The drawing under review shows one solid part. Ordinate dimensions are in mm from its lowest x, y, z. Round coordinates to 2 decimals unless told otherwise and drop trailing zeros. Write each loop counter-clockwise with the first axis right and the second up, starting at its lowest first coordinate (ties: lowest second). Pieces come first, ordered by that corner, then holes. Notation, with made-up numbers: (20, 27.5) - (53, 27.5) arc R4 ccw to (53, 33.5) - close; hole circle Ø10 at (61.25, 73). An arc over 180 degrees is marked (long way). Answer in a Markdown table with one row per item. Add a question column.
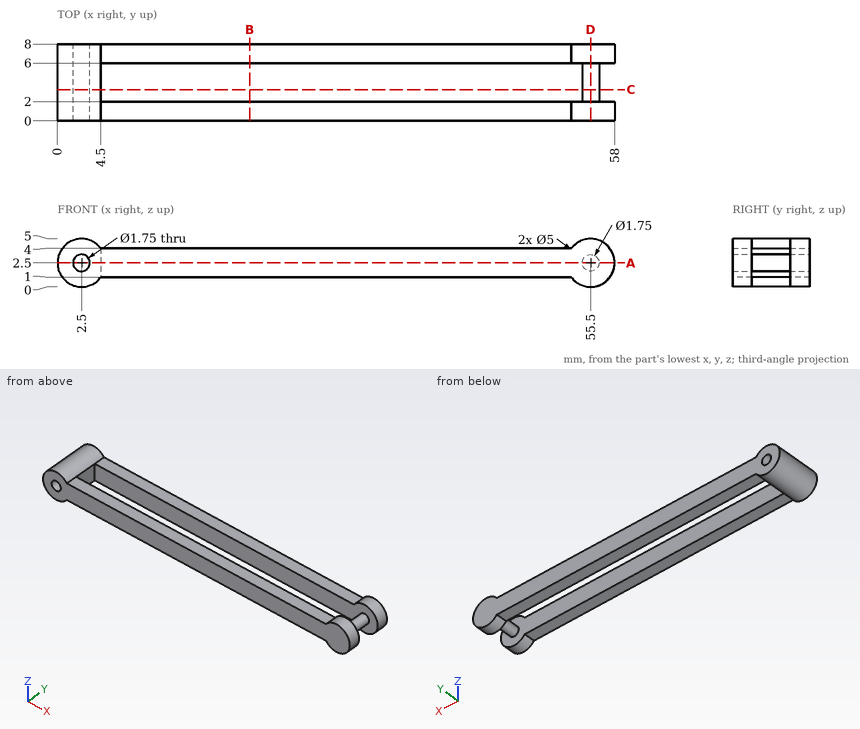
Q1. Add section D-D on x = 55.5. State the section outline as (y, z) points (3 decimals), then the cut area to 3 significant figures.
Q2. Insertion check: pin 1 Ø3 at (x, z) = (48, 4) entering from -Y; pin 2 Ø1 at (x, y) = (31.5, 7) entering from -Z; pin 3 Ø0.6 at (x, y) = (30.5, 6.5) entering from +Z; pin 4 Ø1 at (y, z) = (1, 1) entering from +X. Each pin has a flat end and moves straight along its axis. Give the tip position at first contact, or say it passes through.
Q3. To check wall thickness, follow probe 1 along Z at (x, y) = (2.5, 6.25) (3 decimals); probe 2 along Y at (x, z) = (32.5, 3.95); probe 3 along X at (y, z) = (4.25, 1.8) (3 decimals). State the ranges of each line that lie inside material, in increasing order.
Q4. Add section A-A on z = 2.5. State the section outline as (x, y) points (3 decimals).
Q5. Add section C-C on y = 3.25. State the section outline as (x, z) points (3 decimals).
Q6. Add section B-B on x = 20. State the section outline as (y, z) points.
Answer sheet:
| question | item | result |
|---|---|---|
| 1 | outline | (0, 0) - (2, 0) - (2, 1.625) - (6, 1.625) - (6, 0) - (8, 0) - (8, 5) - (6, 5) - (6, 3.375) - (2, 3.375) - (2, 5) - (0, 5) - close |
| 1 | area | 27.0 mm² |
| 2 | pin 1 | stops at y = 0 |
| 2 | pin 2 | stops at z = 1 |
| 2 | pin 3 | stops at z = 4 |
| 2 | pin 4 | stops at x = 57.79 |
| 3 | probe 1 | z = 0 to 1.625, 3.375 to 5 |
| 3 | probe 2 | y = 0 to 2, 6 to 8 |
| 3 | probe 3 | x = 0.1 to 1.975, 3.025 to 4.5, 54.975 to 56.025 |
| 4 | outline | (0, 0) - (1.625, 0) - (1.625, 8) - (0, 8) - close; (3.375, 0) - (58, 0) - (58, 2) - (56.375, 2) - (56.375, 6) - (58, 6) - (58, 8) - (3.375, 8) - close; hole (4.5, 2) - (54.625, 2) - (54.625, 6) - (4.5, 6) - close |
| 5 | outline | (4.5, 1) - (4.5, 4) arc R2.5 ccw (long way) to start; circle Ø1.75 at (55.5, 2.5); hole circle Ø1.75 at (2.5, 2.5) |
| 6 | outline | (0, 1) - (2, 1) - (2, 4) - (0, 4) - close; (6, 1) - (8, 1) - (8, 4) - (6, 4) - close |
